Model file for the job. Use its own axes, mm. A direction names the side the tool comes from. Round coordinates to 2 decimals unless told otherwise and drop trailing zeros. Loops run counter-clockwise (first coordinate to the right, second up) from the corner with the lowest first, then second, coordinate; pieces in that order, holes last. Notation, with made-up numbers: (20.25, 79.5) - (77.25, 79.5) arc R20 ccw to (77.25, 94.5) - close; hole circle Ø5 at (-38.75, 26). An arc over 180 degrees is marked (long way). Use one line per item in the form item = value.
from build123d import *

# Parameters (mm, degrees)
SKETCH1_W           = 6
SKETCH1_H           = 4.8
BOSS_EXTRUDE1_DEPTH = 2
BOSS_EXTRUDE2_DEPTH = 4
PIN_DEPTH           = 0.25
LPATTERN1_COUNT     = 2
LPATTERN1_PITCH     = 2


with BuildPart() as part:
    # Sketch1 → Boss-Extrude1 (new body)
    with BuildSketch(Plane.XY):
        Rectangle(SKETCH1_W, SKETCH1_H)
    extrude(amount=BOSS_EXTRUDE1_DEPTH)

    # Sketch2 → Boss-Extrude2 (add)
    with BuildSketch(Plane.XY.offset(2)):
        Polygon((-0.5, -2.4), (-0.5, -1.8), (-2.4, -1.8), (-2.4, 1.8), (2.4, 1.8), (2.4, -1.8), (0.5, -1.8), (0.5, -2.4), (3, -2.4), (3, 2.4), (-3, 2.4), (-3, -2.4), align=None)
    extrude(amount=BOSS_EXTRUDE2_DEPTH)

    # Sketch3 → Pin (add, symmetric)
    with BuildSketch(Plane.ZY.offset(1)):
        Polygon((0.25, 5.8), (0.25, -0.35), (5.5, -0.35), (5.5, -0.85), (-0.25, -0.85), (-0.25, 5.8), align=None)
    pin = extrude(amount=PIN_DEPTH, both=True)

    # LPattern1: Pin ×2
    with Locations(*[(i * LPATTERN1_PITCH, 0, 0) for i in range(1, LPATTERN1_COUNT)]):
        add(pin)


solid = part.part
1. Wall check: probe 1 along X at (y, z) = (-0.5, 4); probe 2 along Y at (x, z) = (-0.7, 2.25); probe 3 along X at (y, z) = (-1.25, 2.25). Give the ranges that are in metal, low to high.
Geometry check:
probe_1 = -3 to -2.4, -1.25 to -0.75, 0.75 to 1.25, 2.4 to 3
probe_2 = -2.4 to -1.8, 1.8 to 2.4
probe_3 = -3 to -2.4, 2.4 to 3
2. Pull direction Y, two halves, no side cores. Call faces 1 (the flat face through (1, -2.4, 3)), 2 (the flat face through (-2.4, 0, 4)), 3 (the flat face through (1, -1.8, 4)), 4 (the flat face through (0, 2, 6)): +Y half, -Y half, draft (parallel to the pull), parting line (faces both ways), or undercut.
Geometry check:
face_1 = -Y half
face_2 = undercut
face_3 = undercut
face_4 = draft
3. Cut at C-C, the plane x = 1.85. Give the cut face in (y, z).
Geometry check:
outline = (-2.4, 0) - (2.4, 0) - (2.4, 6) - (1.8, 6) - (1.8, 2) - (-1.8, 2) - (-1.8, 6) - (-2.4, 6) - close
4. Flat gauge pins, fed straight in: pin 1 (2 mm diameter, centred on x = 0.5, z = 2.5, fed in from +Y); pin 2 (0.6 mm diameter, centred on x = -1, y = -0.5, fed in from +Z); pin 3 (0.6 mm diameter, centred on x = 1, y = 4.5, fed in from +Z). Where does each tip first touch, or does it go through?
Geometry check:
pin_1 = 2.4
pin_2 = 5.5
pin_3 = 0.25
5. Tool access for faces 5 (the flat face through (-1, -1.8, 4)), 6 (the flat face through (-3, 0, 3)): list every direction of +Z, -Z, +X, -X, +Y, -Y with a clear straight run to the whole face (end or side of a thin tool).
Geometry check:
face_5 = +Z
face_6 = +Z, -Z, -X, +Y, -Y
6. Cut at A-A, the plane y = 3.75. Give the cut face in (x, z).
Geometry check:
outline = (-1.25, -0.25) - (-0.75, -0.25) - (-0.75, 0.25) - (-1.25, 0.25) - close; (0.75, -0.25) - (1.25, -0.25) - (1.25, 0.25) - (0.75, 0.25) - close
7. Cut at D-D, the plane y = 0.75. Give the cut face in (x, z).
Geometry check:
outline = (-3, 0) - (-1.25, 0) - (-1.25, -0.25) - (-0.75, -0.25) - (-0.75, 0) - (0.75, 0) - (0.75, -0.25) - (1.25, -0.25) - (1.25, 0) - (3, 0) - (3, 6) - (2.4, 6) - (2.4, 2) - (-2.4, 2) - (-2.4, 6) - (-3, 6) - close
8. Cut at B-B, the plane z = 5. Give the cut face in (x, y).
Geometry check:
outline = (-3, -2.4) - (-0.5, -2.4) - (-0.5, -1.8) - (-2.4, -1.8) - (-2.4, 1.8) - (2.4, 1.8) - (2.4, -1.8) - (0.5, -1.8) - (0.5, -2.4) - (3, -2.4) - (3, 2.4) - (-3, 2.4) - close; (-1.25, -0.85) - (-0.75, -0.85) - (-0.75, -0.35) - (-1.25, -0.35) - close; (0.75, -0.85) - (1.25, -0.85) - (1.25, -0.35) - (0.75, -0.35) - close
